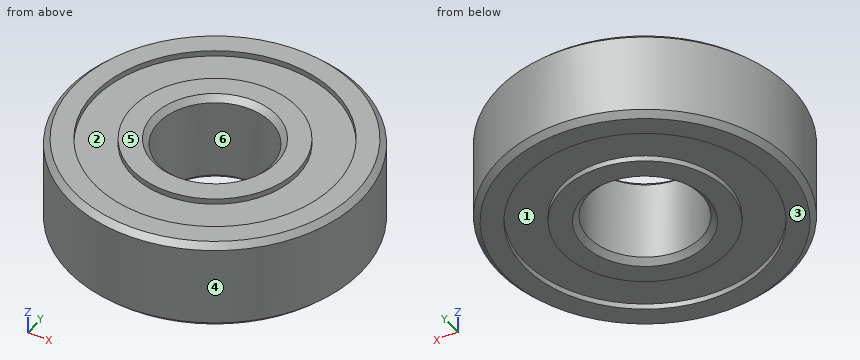
from build123d import *

# Parameters (mm, degrees)
F0_R     = 13
F0_R_2   = 5
F1_DEPTH = 4
F2_R     = 10.7
F2_R_2   = 7.35
F3_DEPTH = 0.5
F4_R     = 10.7
F4_R_2   = 7.35
F5_DEPTH = 0.5
F6_SIZE  = 0.5


with BuildPart() as f1:
    # F0 (on Top) → F1 (new body, symmetric)
    with BuildSketch(Plane.XY):
        Circle(F0_R)
        Circle(F0_R_2, mode=Mode.SUBTRACT)
    extrude(amount=F1_DEPTH, both=True)

    # F2 (on face) → F3 (cut)
    with BuildSketch(Plane(origin=(0, 0, -4), x_dir=(1, 0, 0), z_dir=(0, 0, -1))):
        Circle(F2_R)
        Circle(F2_R_2, mode=Mode.SUBTRACT)
    extrude(amount=-F3_DEPTH, mode=Mode.SUBTRACT)

    # F4 (on face) → F5 (cut)
    with BuildSketch(Plane.XY.offset(4)):
        Circle(F4_R)
        Circle(F4_R_2, mode=Mode.SUBTRACT)
    extrude(amount=-F5_DEPTH, mode=Mode.SUBTRACT)

    # F6
    f6_edges = [f1.edges().sort_by_distance(p)[0] for p in [
        (-13, 0, -4),
        (-13, 0, 4),
        (-5, 0, -4),
        (-5, 0, 4),
    ]]
    chamfer(f6_edges, length=F6_SIZE)


solid = f1.part
The model under review builds one solid part; all positions refer to its coordinate system, in mm. Face numbers are marked on the shaded views. A direction names the side the tool comes from. Round coordinates to 2 decimals unless told otherwise and drop trailing zeros. Loops run counter-clockwise (first coordinate to the right, second up) from the corner with the lowest first, then second, coordinate; pieces in that order, holes last. Notation, with made-up numbers: M -34,46.25 L 0,46.25 A12 cw 0,62.25 Z; hole C 20,42.25 d7. An arc over 180 degrees is marked long. Answer as CSV lines item,"result". Start each with the question number.
Item 1: For the marked faces 1, 2 and 3, list the 3-axis set-ups (+Z, -Z, +X, -X, +Y, -Y) from which the entire face can be reached by the end or side of a thin tool; tool diameter is ignored.
Item 2: Consider section C-C (z = 2). Write out the cut boundary in (x, y), then the cut area to 3 significant figures.
Item 3: Wall thickness on line 1 (Y direction, x = -5.5, z = 3.75); line 2 (Y direction, x = 0, z = 3.65); line 3 (Z direction, x = -8.75, y = 5.25): over which ranges is each line inside the solid? List them lowest first. Write a range as [from, to].
Item 4: Insertion check: P1, Ø6, axis at x = -8.5, y = -1.5, coming from the -Z side; P2, Ø1.5, axis at y = -9, z = 3, coming from the -X side; P3, Ø2, axis at x = 7, z = -3, coming from the +Y side; P4, Ø1, axis at x = -9, y = -3.5, coming from the +Z side. Each pin has a flat end and moves straight along its axis. Give the tip position at first contact, or say it passes through.
Item 5: Mouldability with a two-part tool opening along X and no side actions: class the marked faces 4, 5 and 6 as released by +X, released by -X, zero draft, split by the parting line, or undercut.
Answer:
1,face 1,"-Z"
1,face 2,"+Z"
1,face 3,"-Z, +X, -X, +Y, -Y"
2,outline,"C 0,0 d26; hole C 0,0 d10"
2,area,"452 mm^2"
3,line 1,"y = [-11.5, -9.18], [-4.88, 4.88], [9.18, 11.5]"
3,line 2,"y = [-12.85, -10.7], [-7.35, -5.15], [5.15, 7.35], [10.7, 12.85]"
3,line 3,"z = [-3.5, 3.5]"
4,P1,"stops at z = -4"
4,P2,"stops at x = -10.05"
4,P3,"stops at y = 11.53"
4,P4,"stops at z = 3.5"
5,face 4,"split by the parting line"
5,face 5,"zero draft"
5,face 6,"undercut"
